Can you work these out from the drawing? Everything is in mm from the part's minimum corner. Coordinates: 2 decimals unless noted, no trailing zeros. Loops run counter-clockwise (first coordinate to the right, second up) from the corner with the lowest first, then second, coordinate; pieces in that order, holes last. Notation, with made-up numbers: (61.5, 73) -> (95.5, 73) arc R28 cw to (95.5, 91) -> close; hole circle Ø7 at (-4, -26). An arc over 180 degrees is marked (long way). One line per question, with ' | ' between items.
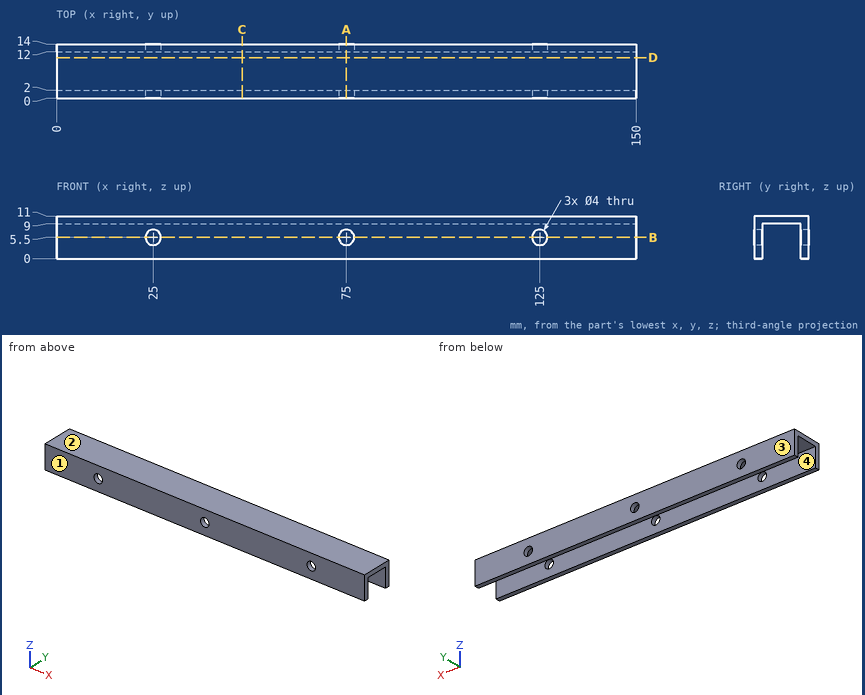
Q1. We'd pull the mould along Y, two halves only. Please class the marked faces 1, 2, 3 and 4: released by +Y, released by -Y, zero draft, split by the parting line, or undercut.
Values follow:
face 1: released by -Y | face 2: zero draft | face 3: released by +Y | face 4: undercut
Q2. Imagine slicing it at D-D on y = 10.5. Write out the boundary of the cut face in (x, z), plus the area to 3 significant figures.
Values follow:
outline: (0, 9) -> (150, 9) -> (150, 11) -> (0, 11) -> close | area: 300 mm2
Q3. For pin 1 (6 mm diameter, centred on y = 7.5, z = 2.5, fed in from +X); pin 2 (1.5 mm diameter, centred on x = 17, y = 5.5, fed in from -Z), each with a flat end and sliding along its axis, tell me the tip position at first contact or that it passes through.
Values follow:
pin 1: passes through | pin 2: stops at z = 9
Q4. Please list where these lines run through material, in increasing order: L1, parallel to Y at x = 29, z = 5.25; L2, parallel to Z at x = 25, y = 13.1; L3, parallel to Z at x = 17.5, y = 9.5. Write a range as [from, to].
Values follow:
L1: y = [0, 2], [12, 14] | L2: z = [0, 3.5], [7.5, 11] | L3: z = [9, 11]
Q5. Imagine slicing it at B-B on z = 5.5. Give the number of separate pieces and of enclosed holes in the cut face, plus the area to 3 significant figures.
Values follow:
separate pieces: 8 | enclosed holes: 0 | area: 552 mm2
Q6. Imagine slicing it at A-A on x = 75. Write out the boundary of the cut face in (y, z), plus the area to 3 significant figures.
Values follow:
outline: (0, 0) -> (2, 0) -> (2, 3.5) -> (0, 3.5) -> close; (0, 7.5) -> (2, 7.5) -> (2, 9) -> (12, 9) -> (12, 7.5) -> (14, 7.5) -> (14, 11) -> (0, 11) -> close; (12, 0) -> (14, 0) -> (14, 3.5) -> (12, 3.5) -> close | area: 48.0 mm2
Q7. Imagine slicing it at C-C on x = 48. Write out the boundary of the cut face in (y, z), plus the area to 3 significant figures.
Values follow:
outline: (0, 0) -> (2, 0) -> (2, 9) -> (12, 9) -> (12, 0) -> (14, 0) -> (14, 11) -> (0, 11) -> close | area: 64.0 mm2
